```python
from build123d import *

# Parameters (mm, degrees)
SKETCH1_W           = 50
SKETCH1_H           = 35
SKETCH1_R           = 9.5
SKETCH1_R_2         = 1.5
BOSS_EXTRUDE3_DEPTH = 6
SKETCH4_W           = 50
SKETCH4_H           = 35
BOSS_EXTRUDE5_DEPTH = 2
BOSS_EXTRUDE6_DEPTH = 55
SKETCH9_R           = 2
CUT_EXTRUDE1_DEPTH  = 8.5
BOSS_EXTRUDE7_DEPTH = 15
FILLET1_R           = 10
FILLET8_R           = 10
SKETCH16_R          = 2
CUT_EXTRUDE2_DEPTH  = 8.5


with BuildPart() as part:
    # Sketch1 → Boss-Extrude3 (new body)
    with BuildSketch(Plane.XY):
        with Locations((25, 17.5)):
            Rectangle(SKETCH1_W, SKETCH1_H)
        with Locations((32.5, 17.5)):
            Circle(SKETCH1_R, mode=Mode.SUBTRACT)
        with Locations((41.692388155, 26.692388155)):
            Circle(SKETCH1_R_2, mode=Mode.SUBTRACT)
        with Locations((41.692388155, 8.307611845)):
            Circle(SKETCH1_R_2, mode=Mode.SUBTRACT)
        with Locations((23.307611845, 8.307611845)):
            Circle(SKETCH1_R_2, mode=Mode.SUBTRACT)
        with Locations((23.307611845, 26.692388155)):
            Circle(SKETCH1_R_2, mode=Mode.SUBTRACT)
    extrude(amount=BOSS_EXTRUDE3_DEPTH)

    # Sketch4 → Boss-Extrude5 (add)
    with BuildSketch(Plane.XY.offset(6)):
        with Locations((25, 17.5)):
            Rectangle(SKETCH4_W, SKETCH4_H)
        with BuildLine():
            ThreePointArc((26.299419693, 26.47083501), (21.186291501, 28.813708499), (23.52916499, 23.700580307))
            ThreePointArc((23.52916499, 23.700580307), (23.763454109, 23.57743344), (23.755822455, 23.312861521))
            ThreePointArc((23.755822455, 23.312861521), (22, 17.5), (23.755822455, 11.687138479))
            ThreePointArc((23.755822455, 11.687138479), (23.763454109, 11.42256656), (23.52916499, 11.299419693))
            ThreePointArc((23.52916499, 11.299419693), (21.186291501, 6.186291501), (26.299419693, 8.52916499))
            ThreePointArc((26.299419693, 8.52916499), (26.42256656, 8.763454109), (26.687138479, 8.755822455))
            ThreePointArc((26.687138479, 8.755822455), (32.5, 7), (38.312861521, 8.755822455))
            ThreePointArc((38.312861521, 8.755822455), (38.57743344, 8.763454109), (38.700580307, 8.52916499))
            ThreePointArc((38.700580307, 8.52916499), (43.813708499, 6.186291501), (41.47083501, 11.299419693))
            ThreePointArc((41.47083501, 11.299419693), (41.236545891, 11.42256656), (41.244177545, 11.687138479))
            ThreePointArc((41.244177545, 11.687138479), (43, 17.5), (41.244177545, 23.312861521))
            ThreePointArc((41.244177545, 23.312861521), (41.236545891, 23.57743344), (41.47083501, 23.700580307))
            ThreePointArc((41.47083501, 23.700580307), (43.813708499, 28.813708499), (38.700580307, 26.47083501))
            ThreePointArc((38.700580307, 26.47083501), (38.57743344, 26.236545891), (38.312861521, 26.244177545))
            ThreePointArc((38.312861521, 26.244177545), (32.5, 28), (26.687138479, 26.244177545))
            ThreePointArc((26.687138479, 26.244177545), (26.42256656, 26.236545891), (26.299419693, 26.47083501))
        make_face(mode=Mode.SUBTRACT)
    extrude(amount=BOSS_EXTRUDE5_DEPTH)

    # Sketch8 → Boss-Extrude6 (add)
    with BuildSketch(Plane(origin=(0, 0, 0), x_dir=(-1, 0, 0), z_dir=(0, 0, -1))):
        with BuildLine():
            Line((-8.5, 35), (-22.740329685, 35))
            Line((-22.740329685, 35), (-22.740329685, 30.367452558))
            ThreePointArc((-22.740329685, 30.367452558), (-20.171344576, 27.9320063), (-18.194683381, 24.99535966))
            Line((-18.194683381, 24.99535966), (-18.194683381, 25))
            Line((-18.194683381, 25), (-8.5, 25))
            Line((-8.5, 25), (-8.5, 10.000000197))
            Line((-8.5, 10.000000197), (-18.197115572, 10.000000197))
            ThreePointArc((-18.197115572, 10.000000197), (-20.17303677, 7.065994176), (-22.740329685, 4.632547442))
            Line((-22.740329685, 4.632547442), (-22.740329685, 0))
            Line((-22.740329685, 0), (-8.5, 0))
            Line((-8.5, 0), (0, 0))
            Line((0, 0), (0, 10.000000197))
            Line((0, 10.000000197), (0, 25))
            Line((0, 25), (0, 35))
            Line((0, 35), (-8.5, 35))
        make_face()
    extrude(amount=BOSS_EXTRUDE6_DEPTH)

    # Sketch9 → Cut-Extrude1 (cut)
    with BuildSketch(Plane.ZY):
        with Locations((-7, 17.5)):
            Circle(SKETCH9_R)
        with Locations((-37, 17.5)):
            Circle(SKETCH9_R)
    extrude(amount=-CUT_EXTRUDE1_DEPTH, mode=Mode.SUBTRACT)

    # Sketch11 → Boss-Extrude7 (add)
    with BuildSketch(Plane(origin=(0, 0, -55), x_dir=(-1, 0, 0), z_dir=(0, 0, -1))):
        Polygon((-8.5, 10.000000197), (-8.5, 35), (0, 35), (0, 0), (-8.5, 0), align=None)
    extrude(amount=BOSS_EXTRUDE7_DEPTH)

    # Fillet1
    fillet1_edges = [part.edges().sort_by_distance(p)[0] for p in [
        (22.740329685, 32.683726279, -55),
    ]]
    fillet(fillet1_edges, radius=FILLET1_R)

    # Fillet8
    fillet8_edges = [part.edges().sort_by_distance(p)[0] for p in [
        (22.740329685, 2.316273721, -55),
    ]]
    fillet(fillet8_edges, radius=FILLET8_R)

    # Sketch16 → Cut-Extrude2 (cut)
    with BuildSketch(Plane(origin=(8.5, 0, 0), x_dir=(0, 0, -1), z_dir=(1, 0, 0))):
        with Locations((62.5, 29.000000197)):
            Circle(SKETCH16_R)
        with Locations((62.5, 6)):
            Circle(SKETCH16_R)
    extrude(amount=-CUT_EXTRUDE2_DEPTH, mode=Mode.SUBTRACT)


solid = part.part
```
Geometry check sheet. Reference: the model listing, model coordinates, mm. A direction names the side the tool comes from. Give positions to 0.01 mm unless a question says otherwise; leave off trailing zeros. Loops run counter-clockwise (first coordinate to the right, second up) from the corner with the lowest first, then second, coordinate; pieces in that order, holes last. Notation, with made-up numbers: (-29.5, -20.75) - (6.5, -20.75) arc R13 ccw to (6.5, 1.25) - close; hole circle Ø8 at (74.5, 83.5). An arc over 180 degrees is marked (long way). Use CSV: the item, a comma, the result in double quotes. Start each with the question number.
Q1. Access from +Z, -Z, +X, -X, +Y, -Y to the whole of each face (thin tool, end or side, straight path). Record for faces 4 (the face through (22.74, 2, -22)), 5 (the face through (4, 18, -70)), 6 (the face through (13, 10, -27)), 7 (the face through (40, 11, 6)).
Q2. Section check B-B, the plane x = 32.5. Record the cut outline in (y, z).
Q3. Section check A-A, the plane z = -62.5. Record the cut outline in (x, y), and give its area (4 significant figures).
Q4. Go/stop test with flat-tipped pins: pin 1 Ø8 at (x, y) = (29, 22) entering from +Z; pin 2 Ø3 at (y, z) = (17.5, -7) entering from -X; pin 3 Ø10.5 at (y, z) = (13, -29.5) entering from +X; pin 4 Ø3 at (x, y) = (25.5, 27.5) entering from -Z. Record where each tip stops, or that it passes through.
Q5. Release check for a two-part mould opening along X. For faces 1 (the face through (4.19, 19.483, -37.26)), 2 (the face through (30.441, 8.226, 2.958)), 3 (the face through (0, 18, -30)) record: +X half, -X half, draft (parallel to the pull), parting line (faces both ways), or undercut.
Q6. Scan lines: probe 1 along Y at (x, z) = (2, -62.5); probe 2 along Y at (x, z) = (32.5, 4.75); probe 3 along Y at (x, z) = (16, -28). Record each from-to range of solid material in increasing order. Write a range as from..to.
Q7. Section check C-C, the plane y = 17.5. Record the cut outline in (x, z), and give its area (3 significant figures).
Findings below:
1,face 4,"-Z, +X, +Y, -Y"
1,face 5,"-Z, +X, -X, +Y, -Y"
1,face 6,"-Z, +X"
1,face 7,"+Z"
2,outline,"(0, 0) - (8, 0) - (8, 6) - (7, 6) - (7, 8) - (0, 8) - close; (27, 0) - (35, 0) - (35, 8) - (28, 8) - (28, 6) - (27, 6) - close"
3,outline,"(0, 0) - (8.5, 0) - (8.5, 4) - (0, 4) - close; (0, 8) - (8.5, 8) - (8.5, 27) - (0, 27) - close; (0, 31) - (8.5, 31) - (8.5, 35) - (0, 35) - close"
3,area,"229.5 mm^2"
4,pin 1,"stops at z = 6"
4,pin 2,"passes through"
4,pin 3,"stops at x = 19.63"
4,pin 4,"stops at z = 0"
5,face 1,"draft"
5,face 2,"undercut"
5,face 3,"-X half"
6,probe 1,"y = 0..4, 8..27, 31..35"
6,probe 2,"y = 0..8, 27..35"
6,probe 3,"y = 0..10, 25..35"
7,outline,"(0, -70) - (8.5, -70) - (8.5, -39) - (0, -39) - close; (0, -35) - (8.5, -35) - (8.5, -9) - (0, -9) - close; (0, -5) - (8.5, -5) - (8.5, 0) - (23, 0) - (23, 6) - (22, 6) - (22, 8) - (0, 8) - close; (42, 0) - (50, 0) - (50, 8) - (43, 8) - (43, 6) - (42, 6) - close"
7,area,"771 mm^2"
